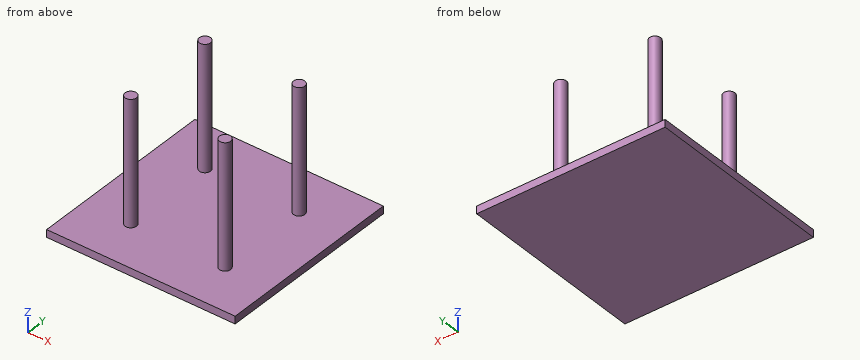
```python
from build123d import *

# Parameters (mm, degrees)
SKETCH_1_W      = 1000
SKETCH_1_H      = 1000
EXTRUDE_1_DEPTH = 40
SKETCH_2_R      = 30
EXTRUDE_2_DEPTH = 700
SKETCH_3_R      = 30
EXTRUDE_3_DEPTH = 700
SKETCH_4_R      = 30
EXTRUDE_4_DEPTH = 700
SKETCH_5_R      = 30
EXTRUDE_5_DEPTH = 700


with BuildPart() as part:
    # 草图1 → 凸台-拉伸1 (new body)
    with BuildSketch(Plane.XY):
        Rectangle(SKETCH_1_W, SKETCH_1_H)
    extrude(amount=EXTRUDE_1_DEPTH)

    # 草图2 → 凸台-拉伸2 (add)
    with BuildSketch(Plane.XY):
        with Locations(Location((-250, -250, 0), (0, 0, 180))):
            Circle(SKETCH_2_R)
    extrude(amount=EXTRUDE_2_DEPTH)

    # 草图3 → 凸台-拉伸3 (add)
    with BuildSketch(Plane.XY):
        with Locations(Location((250, -250, 0), (0, 0, 180))):
            Circle(SKETCH_3_R)
    extrude(amount=EXTRUDE_3_DEPTH)

    # 草图4 → 凸台-拉伸4 (add)
    with BuildSketch(Plane.XY):
        with Locations(Location((-250, 250, 0), (0, 0, 180))):
            Circle(SKETCH_4_R)
    extrude(amount=EXTRUDE_4_DEPTH)

    # 草图5 → 凸台-拉伸5 (add)
    with BuildSketch(Plane.XY):
        with Locations(Location((250, 250, 0), (0, 0, 180))):
            Circle(SKETCH_5_R)
    extrude(amount=EXTRUDE_5_DEPTH)


solid = part.part
```
Here's how the part is built. I have some questions about the finished solid (model axes, mm). Round coordinates to 2 decimals unless told otherwise and drop trailing zeros. Write each loop counter-clockwise with the first axis right and the second up, starting at its lowest first coordinate (ties: lowest second). Pieces come first, ordered by that corner, then holes. Notation, with made-up numbers: M -28.75,64 L 12.25,64 A30 ccw 12.25,100 Z; hole C 4.5,65.5 d7. An arc over 180 degrees is marked long. Answer as CSV lines item,"result". Start each with the question number.
1. Suppose I cut it at A-A on y = -250. Write out the boundary of the cut face in (x, z).
2. I need wall thicknesses on probe 1 along Z at (x, y) = (286, 36.5); probe 2 along X at (y, z) = (256, 301); probe 3 along Y at (x, z) = (-225, 276). Which ranges of each line are inside material? Lowest first, please.
3. Suppose I cut it at D-D on x = -358. Write out the boundary of the cut face in (y, z).
4. I'm going to push a flat-ended pin straight in: pin 1 Ø5 at (x, y) = (156, 25) entering from +Z. Where does the tip first touch, or does it pass through?
5. Suppose I cut it at C-C on z = 183.5. Write out the boundary of the cut face in (x, y).
Check result:
1,outline,"M -500,0 L 500,0 L 500,40 L 280,40 L 280,700 L 220,700 L 220,40 L -220,40 L -220,700 L -280,700 L -280,40 L -500,40 Z"
2,probe 1,"z = 0 to 40"
2,probe 2,"x = -279.39 to -220.61, 220.61 to 279.39"
2,probe 3,"y = -266.58 to -233.42, 233.42 to 266.58"
3,outline,"M -500,0 L 500,0 L 500,40 L -500,40 Z"
4,pin 1,"stops at z = 40"
5,outline,"C -250,-250 d60; C -250,250 d60; C 250,-250 d60; C 250,250 d60"
